Verification items for the finished model (mm, model axes). Round coordinates to 2 decimals unless told otherwise and drop trailing zeros. Order: outer loops, then holes, each group sorted by start corner. A loop starts at its lowest first (then second) coordinate and runs counter-clockwise, first axis right, second up. Notation, with made-up numbers: (35.5, 83.5) -> (39.5, 83.5) arc R30 ccw to (39.5, 108.5) -> close; hole circle Ø7 at (-40, -16). An arc over 180 degrees is marked (long way). Return JSON: item names as keys, results as strings. Group by question number.
Item 1: Sectioned sample at A-A on x = 0. Record the cut outline in (y, z) (3 decimals).
Item 2: Scan lines: probe 1 along Z at (x, y) = (0, 0.65) (3 decimals); probe 2 along X at (y, z) = (0.95, -1); probe 3 along Z at (x, y) = (-1.5, 1.45) (3 decimals). Record each from-to range of solid material in increasing order. Write a range as from..to.
Item 3: Sectioned sample at C-C on y = 0.45. Record the cut outline in (x, z) (3 decimals).
Item 4: Sectioned sample at B-B on z = -1.5. Record the cut outline in (x, y).
```python
from build123d import *

# Parameters (mm, degrees)
SKETCH1_W           = 10.24
SKETCH1_H           = 34.73
BOSS_EXTRUDE1_DEPTH = 1.5
CHAMFER1_SIZE       = 0.5
CHAMFER2_SIZE       = 1
SKETCH2_R           = 1.75
CUT_EXTRUDE1_DEPTH  = 2.5


with BuildPart() as part:
    # Sketch1 → Boss-Extrude1 (new body)
    with BuildSketch(Plane(origin=(0, 0, 0), x_dir=(1, 0, 0), z_dir=(0, 1, 0))):
        Rectangle(SKETCH1_W, SKETCH1_H)
    extrude(amount=BOSS_EXTRUDE1_DEPTH)

    # Chamfer1
    chamfer1_edges = [part.edges().sort_by_distance(p)[0] for p in [
        (-5.12, 0.75, -17.365),
        (5.12, 0.75, -17.365),
    ]]
    chamfer(chamfer1_edges, length=CHAMFER1_SIZE)

    # Chamfer2
    chamfer2_edges = [part.edges().sort_by_distance(p)[0] for p in [
        (5.12, 0.75, 17.365),
        (-5.12, 0.75, 17.365),
    ]]
    chamfer(chamfer2_edges, length=CHAMFER2_SIZE)

    # Sketch2 → Cut-Extrude1 (cut, through all)
    with BuildSketch(Plane(origin=(0, 1.5, 0), x_dir=(1, 0, 0), z_dir=(0, 1, 0))):
        with Locations((0, 0.515)):
            Circle(SKETCH2_R)
    extrude(amount=-CUT_EXTRUDE1_DEPTH, mode=Mode.SUBTRACT)


solid = part.part
```
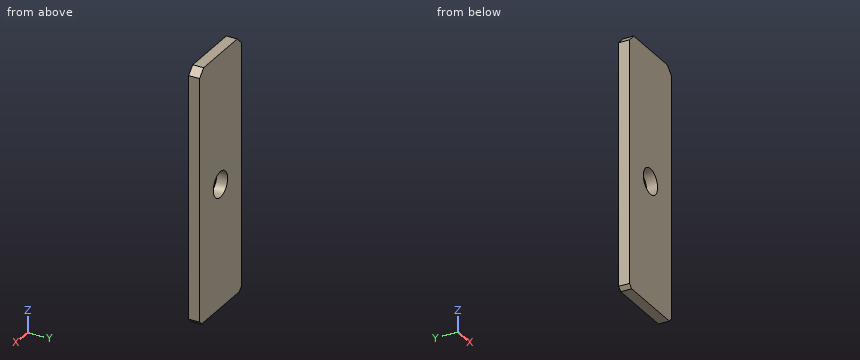
Recorded:
{
 "1": {"outline": "(0, -17.365) -> (1.5, -17.365) -> (1.5, -2.265) -> (0, -2.265) -> close; (0, 1.235) -> (1.5, 1.235) -> (1.5, 17.365) -> (0, 17.365) -> close"},
 "2": {"probe 1": "-17.365..-2.265, 1.235..17.365", "probe 2": "-5.12..-1.68, 1.68..5.12", "probe 3": "-17.365..-1.416, 0.386..17.365"},
 "3": {"outline": "(-5.12, -16.865) -> (-4.62, -17.365) -> (4.62, -17.365) -> (5.12, -16.865) -> (5.12, 16.365) -> (4.12, 17.365) -> (-4.12, 17.365) -> (-5.12, 16.365) -> close; hole circle Ø3.5 at (0, -0.515)"},
 "4": {"outline": "(-5.12, 0) -> (-1.45, 0) -> (-1.45, 1.5) -> (-5.12, 1.5) -> close; (1.45, 0) -> (5.12, 0) -> (5.12, 1.5) -> (1.45, 1.5) -> close"}
}
